Autodesk Inventor part; units mm, degrees
ref_plane "YZ Plane" through (0, 0, 0) normal (1, 0, 0) x (0, 1, 0)
ref_plane "XZ Plane" through (0, 0, 0) normal (0, 1, 0) x (-1, 0, 0)
ref_plane "XY Plane" through (0, 0, 0) normal (0, 0, 1) x (1, 0, 0)
sketch "Skizze2" plane through (0, 0, 0) normal (0, 0, 1) x (1, 0, 0)
  line L0 (0, 18) -> (35, 18)
  line L1 (35, 18) -> (35, 0)
  line L2 (35, 0) -> (0, 0)
  line L3 (0, 0) -> (0, 18)
  dimension "d12" = 18
  dimension "d13" = 35
extrude "Grobblech2" add sketch "Skizze2" along normal blind 0.5
sketch "Skizze3" plane through (0, 17.5, 0) normal (0, 1, 0) x (-1, 0, 0)
  line L0 (-35, 0) -> (0, 0)
  line L1 (0, 0) -> (0, 18)
  line L2 (0, 18) -> (-35, 18)
  line L3 (-35, 18) -> (-35, 0)
edge flange "Lasche1" height 18 angle 90 thickness 0.5 bend radius 0.5 thickness toward (0, 1, 0) relief tear relief width 0.5 relief depth 0.25 edges at (17.5, 18, 0.5) wall of the first edge with corners at (35, 17.5, 0) (0, 17.5, 0) (0, 17.5, 18) (35, 17.5, 18)
bend "Biegung1"
corner "Ecke1"
sketch "Skizze4" plane through (35, 0.5, 0) normal (0, -1, 0) x (1, 0, 0)
  line L0 (-35, 0) -> (0, 0)
  line L1 (0, 0) -> (0, 18)
  line L2 (0, 18) -> (-35, 18)
  line L3 (-35, 18) -> (-35, 0)
edge flange "Lasche2" height 18 angle 90 thickness 0.5 bend radius 0.5 thickness toward (0, -1, 0) relief tear relief width 0.5 relief depth 0.25 edges at (17.5, 0, 0.5) wall of the first edge with corners at (0, 0.5, 0) (35, 0.5, 0) (35, 0.5, 18) (0, 0.5, 18)
bend "Biegung2"
corner "Ecke2"
sketch "Skizze5" plane through (35, 17.5, 17.5) normal (0, 0, 1) x (1, 0, 0)
  line L0 (-35, 0) -> (0, 0)
  line L1 (0, 0) -> (0, 15.5)
  line L2 (0, 15.5) -> (-35, 15.5)
  line L3 (-35, 15.5) -> (-35, 0)
edge flange "Lasche3" height 15.5 angle 90 thickness 0.5 bend radius 0.5 thickness toward (0, 0, 1) relief tear relief width 0.5 relief depth 0.25 edges at (17.5, 18, 18) wall of the first edge with corners at (0, 17.5, 17.5) (35, 17.5, 17.5) (35, 33, 17.5) (0, 33, 17.5)
bend "Biegung3"
corner "Ecke3"
sketch "Skizze6" plane through (0, 0.5, 17.5) normal (0, 0, 1) x (1, 0, 0)
  line L0 (35, 0) -> (0, 0)
  line L1 (0, 0) -> (0, -15.5)
  line L2 (0, -15.5) -> (35, -15.5)
  line L3 (35, -15.5) -> (35, 0)
edge flange "Lasche4" height 15.5 angle 90 thickness 0.5 bend radius 0.5 thickness toward (0, 0, 1) relief tear relief width 0.5 relief depth 0.25 edges at (17.5, 0, 18) wall of the first edge with corners at (35, 0.5, 17.5) (0, 0.5, 17.5) (0, -15, 17.5) (35, -15, 17.5)
bend "Biegung4"
corner "Ecke4"
sketch "Skizze7" plane through (0, 0, 1) normal (0, -1, 0) x (1, 0, 0)
  line L0 (35, -1) -> (21, -1)
  line L1 (21, -1) -> (21, 7)
  line L2 (21, 7) -> (35, 7)
  line L3 (35, 7) -> (35, -1)
  line L4 (35, -1) -> (0, -1)
  dimension "d55" = 8
  dimension "d56" = 14
extrude "Ausschneiden1" cut sketch "Skizze7" against normal up to surface (18 mm away)
sketch "Skizze8" plane through (0, 0, 0) normal (0, 0, -1) x (-1, 0, 0)
  line L0 (-21, 17) -> (-21, 1)
  line L1 (-21, 1) -> (0, 1)
  line L2 (0, 17) -> (0, 1)
  line L3 (0, 17) -> (-21, 17)
  line L4 (0, 9) -> (-30.5159, 9) construction
  line L5 (-35, -15) -> (0, -15)
  line L6 (-17.5, -15) -> (-17.5, 33) construction
  line L7 (0, 33) -> (-35, 33)
  point P0 (0, 0)
  point P1 (-30, 28)
  point P2 (-5, 28)
  point P3 (-30, -10)
  point P4 (-5, -10)
  dimension "d59" = 25
  dimension "d60" = 38
  dimension "d61" = 25
  dimension "d62" = 38
hole "Bohrung1" at (30, 28, 0) at (5, 28, 0) at (30, -10, 0) at (5, -10, 0) direction (0, 0, 1) diameter 4.5 depth 18
sketch "Skizze9" plane through (0, 0, 0) normal (0, 0, -1) x (-1, 0, 0)
  line L0 (0, 17) -> (0, 1)
  point P0 (0, 0)
  point P1 (-8, 8.1851)
  point P2 (-16, 8.1851)
  dimension "d70" = 8
  dimension "d71" = 8
hole "Bohrung2" at (8, 8.1851, 0) at (16, 8.1851, 0) direction (0, 0, 1) diameter 3 end through all
equation "\"d57\" = Stärke"
equation "\"d68\" = Stärke"
equation "\"d14\" = Stärke"
equation "\"d15\" = BreiteBiegungsfreistellung"
equation "\"d16\" = TiefeBiegungsfreistellung"
equation "\"d17\" = MinimalRest"
equation "\"d18\" = Übergangsradius"
equation "\"d21\" = Biegeradius"
equation "\"d22\" = GrößeEckenfreistellung"
equation "\"d23\" = Abstandsgröße"
equation "\"d24\" = JacobiRadiusGröße"
equation "\"d25\" = BreiteBiegungsfreistellung"
equation "\"d26\" = TiefeBiegungsfreistellung"
equation "\"d27\" = MinimalRest"
equation "\"d28\" = Übergangsradius"
equation "\"d31\" = Biegeradius"
equation "\"d32\" = GrößeEckenfreistellung"
equation "\"d33\" = Abstandsgröße"
equation "\"d34\" = JacobiRadiusGröße"
equation "\"d35\" = BreiteBiegungsfreistellung"
equation "\"d36\" = TiefeBiegungsfreistellung"
equation "\"d37\" = MinimalRest"
equation "\"d38\" = Übergangsradius"
equation "\"d41\" = Biegeradius"
equation "\"d42\" = GrößeEckenfreistellung"
equation "\"d43\" = Abstandsgröße"
equation "\"d44\" = JacobiRadiusGröße"
equation "\"d45\" = BreiteBiegungsfreistellung"
equation "\"d46\" = TiefeBiegungsfreistellung"
equation "\"d47\" = MinimalRest"
equation "\"d48\" = Übergangsradius"
equation "\"d51\" = Biegeradius"
equation "\"d52\" = GrößeEckenfreistellung"
equation "\"d53\" = Abstandsgröße"
equation "\"d54\" = JacobiRadiusGröße"
equation "\"Biegeradius\" = Stärke"
equation "\"BreiteBiegungsfreistellung\" = Stärke"
equation "\"TiefeBiegungsfreistellung\" = 0.5 * Stärke"
equation "\"GrößeEckenfreistellung\" = 4 * Stärke"
equation "\"MinimalRest\" = 2 * Stärke"
equation "\"Übergangsradius\" = Biegeradius"
equation "\"JacobiRadiusGröße\" = Biegeradius"
equation "\"Abstandsgröße\" = Stärke"
properties part number "Bügelbefestigung" material "Stahl, galvanisiert"
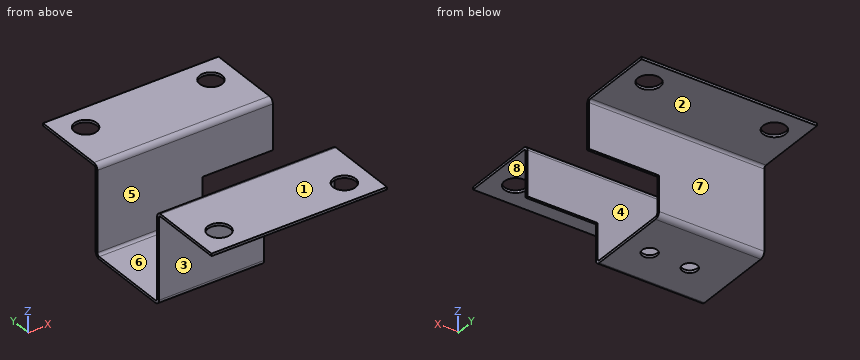
Geometry check sheet. Reference: the model listing, model coordinates, mm. Face numbers are marked on the shaded views. A direction names the side the tool comes from. Coordinates: 2 decimals unless noted, no trailing zeros. Order: outer loops, then holes, each group sorted by start corner. A loop starts at its lowest first (then second) coordinate and runs counter-clockwise, first axis right, second up. Notation, with made-up numbers: (30, 58.5) - (75, 58.5) arc R22 ccw to (75, 88.5) - close; hole circle Ø6 at (61.25, 68.5). An arc over 180 degrees is marked (long way). Answer in a Markdown table with one row per item. Add a question column.
1. Section check A-A (x = 5). Enter the section's corners in (y, z).
2. Section check C-C (x = 33). Enter the section's corners in (y, z).
3. Section check B-B (z = 1.5). Enter the section's corners in (x, y).
4. Material ranges on L1, parallel to X at y = 28, z = 17.65; L2, parallel to Y at x = 17, z = 8; L3, parallel to Y at x = 5, z = 17.75, recorded low to high. Write a range as [from, to].
5. Draft check along Y on the marked faces 5, 6, 7 and 8. Enter one of: +Y half, -Y half, draft (parallel to the pull), parting line (faces both ways), or undercut.
6. Section check D-D (y = 28). Enter the section's corners in (x, z), plus the area to 3 significant figures.
7. Gauge pin test, flat ends, axial feed: pin 1 Ø4 at (x, z) = (10.5, 2.5) entering from -Y; pin 2 Ø1.5 at (x, y) = (14.5, -4) entering from -Z; pin 3 Ø5 at (x, z) = (12.5, 10.5) entering from +Y. Record the tip position at first contact, or that the pin passes through.
8. Access from +Z, -Z, +X, -X, +Y, -Y to the whole of each face (thin tool, end or side, straight path). Record for the marked faces 1, 2, 3 and 4.
Data:
| question | item | result |
|---|---|---|
| 1 | outline | (-15, 17.5) - (-12.25, 17.5) - (-12.25, 18) - (-15, 18) - close; (-7.75, 17.5) - (-0.5, 17.5) arc R0.5 cw to (0, 17) - (0, 1) arc R1 ccw to (1, 0) - (17, 0) arc R1 ccw to (18, 1) - (18, 17) arc R0.5 cw to (18.5, 17.5) - (25.75, 17.5) - (25.75, 18) - (18.5, 18) arc R1 ccw to (17.5, 17) - (17.5, 1) arc R0.5 cw to (17, 0.5) - (1, 0.5) arc R0.5 cw to (0.5, 1) - (0.5, 17) arc R1 ccw to (-0.5, 18) - (-7.75, 18) - close; (30.25, 17.5) - (33, 17.5) - (33, 18) - (30.25, 18) - close |
| 2 | outline | (-15, 17.5) - (-0.5, 17.5) arc R0.5 cw to (0, 17) - (0, 8) - (0.5, 8) - (0.5, 17) arc R1 ccw to (-0.5, 18) - (-15, 18) - close; (17.5, 8) - (18, 8) - (18, 17) arc R0.5 cw to (18.5, 17.5) - (33, 17.5) - (33, 18) - (18.5, 18) arc R1 ccw to (17.5, 17) - close |
| 3 | outline | (0, 0) - (21, 0) - (21, 0.5) - (0, 0.5) - close; (0, 17.5) - (21, 17.5) - (21, 18) - (0, 18) - close |
| 4 | L1 | x = [0, 2.75], [7.25, 27.75], [32.25, 35] |
| 4 | L2 | y = [0, 0.5], [17.5, 18] |
| 4 | L3 | y = [-15, -12.25], [-7.75, 0.16], [17.84, 25.75], [30.25, 33] |
| 5 | face 5 | undercut |
| 5 | face 6 | undercut |
| 5 | face 7 | +Y half |
| 5 | face 8 | draft |
| 6 | outline | (0, 17.5) - (2.75, 17.5) - (2.75, 18) - (0, 18) - close; (7.25, 17.5) - (27.75, 17.5) - (27.75, 18) - (7.25, 18) - close; (32.25, 17.5) - (35, 17.5) - (35, 18) - (32.25, 18) - close |
| 6 | area | 13.0 mm² |
| 7 | pin 1 | stops at y = 0 |
| 7 | pin 2 | stops at z = 17.5 |
| 7 | pin 3 | stops at y = 18 |
| 8 | face 1 | +Z, +X, -X, +Y, -Y |
| 8 | face 2 | -Z, +X, -X, +Y |
| 8 | face 3 | -Z, +X, -X, -Y |
| 8 | face 4 | +Z, +X, -X |
